Input: dimensioned drawing with shaded views. Units: mm. Origin: part minimum x, y, z. A direction names the side the tool comes from. Give positions to 0.01 mm unless a question says otherwise; leave off trailing zeros. Loops run counter-clockwise (first coordinate to the right, second up) from the corner with the lowest first, then second, coordinate; pieces in that order, holes last. Notation, with made-up numbers: (-16.75, 12.25) -> (5.25, 12.25) arc R34 cw to (5.25, 50.25) -> close; hole circle Ø11 at (-14, 62.5). An arc over 180 degrees is marked (long way). Answer in a Markdown table with one row per item. Add a question column.
1) Access query for the marked faces 1, 2 and 3. Directions: +Z, -Z, +X, -X, +Y, -Y. A direction counts if a zero-diameter tool reaches every point of the face in a straight line with its end or side. Return the directions, or none.
2) First-contact query: P1, Ø2, axis at x = 27.5, z = 10, coming from the -Y side; P2, Ø1.5, axis at y = 2, z = 49.5, coming from the +X side; P3, Ø9, axis at x = 110, z = 10, coming from the +Y side. Flat tips, straight axial feed; report the tip coordinate or a pass-through.
3) Section query A-A (y = 6). Return the cut outline in (x, z).
4) Line query: line 1 (Z direction, x = 110, y = 5.75); line 2 (X direction, y = 9.25, z = 14); line 3 (X direction, y = 10.25, z = 7.5). Output: solid intervals per line, ascending. Write a range as from..to.
5) Section query B-B (z = 27). Return the cut outline in (x, y), plus the area to 3 significant figures.
6) Section query C-C (x = 69.5). Return the cut outline in (y, z), plus the area to 3 significant figures.
7) Draft query along X for the marked faces 4, 5 and 6. Return one class per face: +X half, -X half, draft (parallel to the pull), parting line (faces both ways), or undercut.
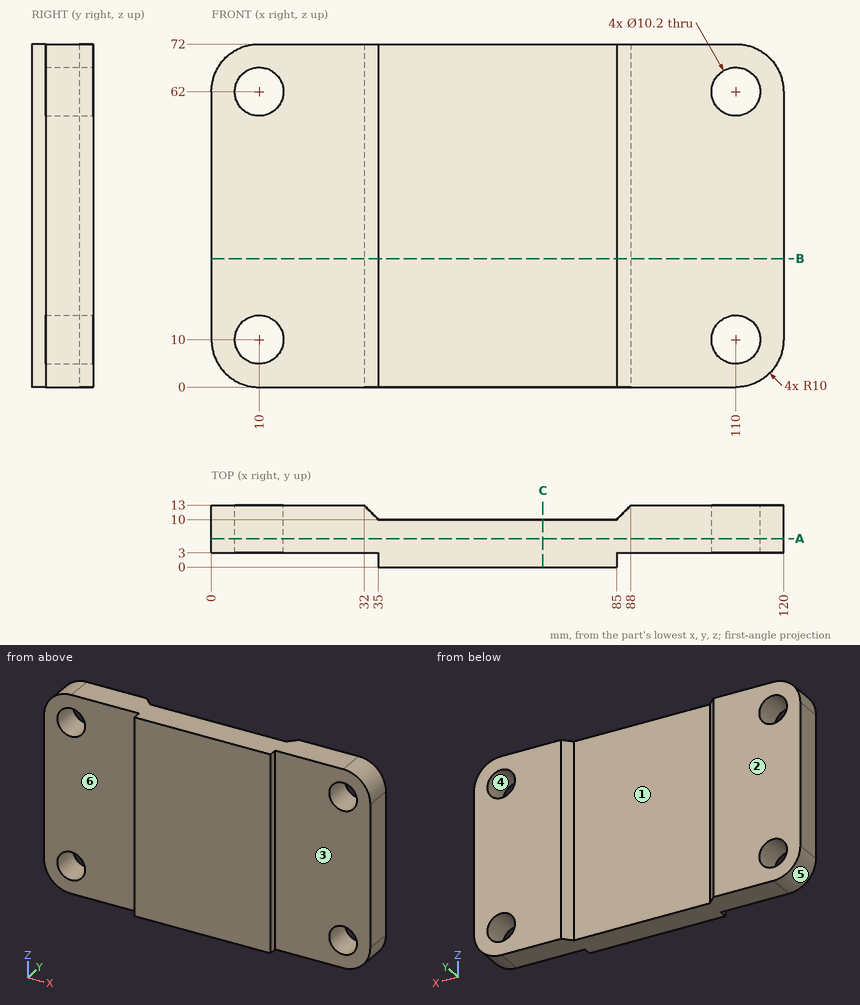
Evaluation:
| question | item | result |
|---|---|---|
| 1 | face 1 | +Z, -Z, +Y |
| 1 | face 2 | +Z, -Z, +X, -X, +Y |
| 1 | face 3 | +Z, -Z, +X, -Y |
| 2 | P1 | y = 3 |
| 2 | P2 | x = 85 |
| 2 | P3 | through |
| 3 | outline | (0, 10) arc R10 ccw to (10, 0) -> (110, 0) arc R10 ccw to (120, 10) -> (120, 62) arc R10 ccw to (110, 72) -> (10, 72) arc R10 ccw to (0, 62) -> close; hole circle Ø10.2 at (10, 10); hole circle Ø10.2 at (10, 62); hole circle Ø10.2 at (110, 10); hole circle Ø10.2 at (110, 62) |
| 4 | line 1 | 0..4.9, 15.1..56.9, 67.1..72 |
| 4 | line 2 | 0..6.84, 13.16..106.84, 113.16..120 |
| 4 | line 3 | 0.32..5.55, 14.45..34.75, 85.25..105.55, 114.45..119.68 |
| 5 | outline | (0, 3) -> (35, 3) -> (35, 0) -> (85, 0) -> (85, 3) -> (120, 3) -> (120, 13) -> (88, 13) -> (85, 10) -> (35, 10) -> (32, 13) -> (0, 13) -> close |
| 5 | area | 1,190 mm² |
| 6 | outline | (0, 0) -> (10, 0) -> (10, 72) -> (0, 72) -> close |
| 6 | area | 720 mm² |
| 7 | face 4 | undercut |
| 7 | face 5 | -X half |
| 7 | face 6 | draft |
